```python
from build123d import *
from OCP.BRepFilletAPI import BRepFilletAPI_MakeChamfer

# Parameters (mm, degrees)
ESQUISSE1_R             = 0.8
ESQUISSE1_R_2           = 1.5
BOSS_EXTRU_1_DEPTH      = 3.3
BOSS_EXTRU_2_DEPTH      = 1.4
BOSS_EXTRU_2_DEPTH_BACK = 4.7
ESQUISSE2_R             = 3.5
CHANFREIN1_SIZE         = 5
CHANFREIN1_SIZE2        = 1.339745962
CHANFREIN3_SIZE         = 1


with BuildPart() as part:
    # Esquisse1 → Boss.-Extru.1 (new body)
    with BuildSketch(Plane.XY):
        with BuildLine():
            Line((0, -7.1), (29, -4.1))
            ThreePointArc((29, -4.1), (33.1, 0), (29, 4.1))
            Line((29, 4.1), (0, 7.1))
            ThreePointArc((0, 7.1), (-7.1, 0), (0, -7.1))
        make_face()
        with Locations((29, 0)):
            Circle(ESQUISSE1_R, mode=Mode.SUBTRACT)
        with Locations((26, 0)):
            Circle(ESQUISSE1_R, mode=Mode.SUBTRACT)
        with Locations((23, 0)):
            Circle(ESQUISSE1_R, mode=Mode.SUBTRACT)
        with Locations((20, 0)):
            Circle(ESQUISSE1_R, mode=Mode.SUBTRACT)
        with Locations((17, 0)):
            Circle(ESQUISSE1_R, mode=Mode.SUBTRACT)
        Circle(ESQUISSE1_R_2, mode=Mode.SUBTRACT)
    extrude(amount=BOSS_EXTRU_1_DEPTH)

    # Esquisse2 → Boss.-Extru.2 (add, two sides: drawn at the far end of the back side and taken through both)
    with BuildSketch(Plane.XY.offset(3.3).offset(-BOSS_EXTRU_2_DEPTH_BACK)):
        with BuildLine():
            Line((0, -7.1), (11, -5.962068966))
            Line((11, -5.962068966), (11, 5.962068966))
            Line((11, 5.962068966), (0, 7.1))
            ThreePointArc((0, 7.1), (-7.1, 0), (0, -7.1))
        make_face()
        Circle(ESQUISSE2_R, mode=Mode.SUBTRACT)
    extrude(amount=BOSS_EXTRU_2_DEPTH + BOSS_EXTRU_2_DEPTH_BACK)

    # Chanfrein1: one chamfer whose edges measure the first distance from different faces: ONE call of the kernel's chamfer builder (chamfer() names one face for all edges)
    chanfrein1_edges_1 = [part.edges().sort_by_distance(p)[0] for p in [
        (11, 0, -1.4),
    ]]
    chanfrein1_side_1 = [part.faces().sort_by_distance(p)[0] for p in [
        (5.476327604, -6.302201317, -1.4),
    ]]
    chanfrein1_edges_2 = [part.edges().sort_by_distance(p)[0] for p in [
        (11, 0, 4.7),
    ]]
    chanfrein1_side_2 = [part.faces().sort_by_distance(p)[0] for p in [
        (5.476327604, -6.302201317, 4.7),
    ]]
    chanfrein1 = BRepFilletAPI_MakeChamfer(part.part.solid().wrapped)
    for e in chanfrein1_edges_1:
        chanfrein1.Add(CHANFREIN1_SIZE, CHANFREIN1_SIZE2, e.wrapped, chanfrein1_side_1[0].wrapped)  # the first distance lies on this face
    for e in chanfrein1_edges_2:
        chanfrein1.Add(CHANFREIN1_SIZE, CHANFREIN1_SIZE2, e.wrapped, chanfrein1_side_2[0].wrapped)  # the first distance lies on this face
    add(Compound.cast(chanfrein1.Shape()), mode=Mode.REPLACE)

    # Chanfrein3
    chanfrein3_edges = [part.edges().sort_by_distance(p)[0] for p in [
        (3, -6.789655172, 4.7),
    ]]
    chamfer(chanfrein3_edges, length=CHANFREIN3_SIZE)
    chanfrein3_2_edges = [part.edges().sort_by_distance(p)[0] for p in [
        (3, -6.789655172, -1.4),
    ]]
    chamfer(chanfrein3_2_edges, length=CHANFREIN3_SIZE)
    chanfrein3_3_edges = [part.edges().sort_by_distance(p)[0] for p in [
        (3, 6.789655172, 4.7),
    ]]
    chamfer(chanfrein3_3_edges, length=CHANFREIN3_SIZE)
    chanfrein3_4_edges = [part.edges().sort_by_distance(p)[0] for p in [
        (3, 6.789655172, -1.4),
    ]]
    chamfer(chanfrein3_4_edges, length=CHANFREIN3_SIZE)
    chanfrein3_5_edges = [part.edges().sort_by_distance(p)[0] for p in [
        (-7.1, 0, 4.7),
    ]]
    chamfer(chanfrein3_5_edges, length=CHANFREIN3_SIZE)
    chanfrein3_6_edges = [part.edges().sort_by_distance(p)[0] for p in [
        (-7.1, 0, -1.4),
    ]]
    chamfer(chanfrein3_6_edges, length=CHANFREIN3_SIZE)


solid = part.part
```
Work out the finished part from the listing and answer in its coordinate system (mm). A direction names the side the tool comes from. Give positions to 0.01 mm unless a question says otherwise; leave off trailing zeros. Order: outer loops, then holes, each group sorted by start corner. A loop starts at its lowest first (then second) coordinate and runs counter-clockwise, first axis right, second up.
1. Straight lines are drawn through the part: L1, parallel to Y at x = 0, z = 1.1; L2, parallel to Z at x = 22.5, y = -2.25; L3, parallel to Y at x = 0, z = 4.05. For each, find the intervals that lie inside material, in ascending order.
Result sheet:
L1: y = -7.1 to -1.5, 1.5 to 7.1
L2: z = 0 to 3.3
L3: y = -6.75 to -3.5, 3.5 to 6.75
2. Section D-D, the plane x = 2 is taken. Determine the outline of the cut face in (y, z).
Result sheet:
outline: (-6.89, -0.4) - (-5.89, -1.4) - (-2.87, -1.4) - (-2.87, 0) - (2.87, 0) - (2.87, -1.4) - (5.89, -1.4) - (6.89, -0.4) - (6.89, 3.7) - (5.89, 4.7) - (2.87, 4.7) - (2.87, 3.3) - (-2.87, 3.3) - (-2.87, 4.7) - (-5.89, 4.7) - (-6.89, 3.7) - close
3. The mould has two halves that part along X. Classify faces 4 (the flat face through (22, 0, 3.3)), 5 (the cylindrical face through (3.233, -1.341, -0.71)), 6 (the flat face through (3.66, -6.21, -0.91)): released by +X, released by -X, zero draft, split by the parting line, or undercut.
Result sheet:
face 4: zero draft
face 5: undercut
face 6: released by +X
4. For faces 1 (the flat face through (22, 0, 0)), 2 (the cylindrical face through (3.233, -1.341, 3.99)), 3 (the flat face through (3.67, -6.23, 4.19)), determine the directions among +Z, -Z, +X, -X, +Y, -Y from which every point of the face is accessible in a straight line to the end or side of a thin tool.
Result sheet:
face 1: -Z, +X, +Y, -Y
face 2: +Z
face 3: +Z, +X, -Y
5. Section C-C, the plane x = 20 is taken. Determine the outline of the cut face in (y, z), and give its area (3 significant figures).
Result sheet:
outline: (-5.03, 0) - (-0.8, 0) - (-0.8, 3.3) - (-5.03, 3.3) - close; (0.8, 0) - (5.03, 0) - (5.03, 3.3) - (0.8, 3.3) - close
area: 27.9 mm2
6. Section B-B, the plane x = 26 is taken. Determine the outline of the cut face in (y, z).
Result sheet:
outline: (-4.41, 0) - (-0.8, 0) - (-0.8, 3.3) - (-4.41, 3.3) - close; (0.8, 0) - (4.41, 0) - (4.41, 3.3) - (0.8, 3.3) - close
7. Section A-A, the plane z = 1.5 is taken. Determine the outline of the cut face in (x, y), and give its area (3 significant figures).
Result sheet:
outline: (0, -7.1) - (29, -4.1) arc R4.1 ccw to (29, 4.1) - (0, 7.1) arc R7.1 ccw to start; hole circle Ø3 at (0, 0); hole circle Ø1.6 at (17, 0); hole circle Ø1.6 at (20, 0); hole circle Ø1.6 at (23, 0); hole circle Ø1.6 at (26, 0); hole circle Ø1.6 at (29, 0)
area: 413 mm2
8. Each of these flat-tipped pins is pushed along its axis until it touches: P1, Ø5.5, axis at x = 0, y = 0, coming from the -Z side; P2, Ø5, axis at x = 18.5, y = -4, coming from the +Z side; P3, Ø1.3, axis at x = 20, y = 0, coming from the -Z side (1 decimal); P4, Ø1.5, axis at y = 3.5, z = 3, coming from the -X side. Where does it stop, or does it pass through?
Result sheet:
P1: stops at z = 0
P2: stops at z = 3.3
P3: passes through
P4: stops at x = -6.55
